Autodesk Inventor part; units mm, degrees
ref_plane "YZ Plane" through (0, 0, 0) normal (1, 0, 0) x (0, 1, 0)
ref_plane "XZ Plane" through (0, 0, 0) normal (0, 1, 0) x (-1, 0, 0)
ref_plane "XY Plane" through (0, 0, 0) normal (0, 0, 1) x (1, 0, 0)
sketch "Sketch1" plane through (0, 0, 0) normal (0, 0, 1) x (1, 0, 0)
  line L0 (0, 0) -> (14.9, 0)
  line L1 (14.9, 0) -> (14.9, 2.75)
  line L2 (14.9, 2.75) -> (12, 2.75)
  line L3 (0, 0) -> (0, 1.5)
  line L4 (0, 1.5) -> (12, 1.5)
  line L5 (12, 1.5) -> (12, 2.75)
  dimension "d0" = 14.9
  dimension "d1" = 2.75
  dimension "d2" = 2.9
  dimension "d3" = 1.5
revolve "Revolution1" add sketch "Sketch1" angle 360 about axis through (0, 0, 0) along (1, 0, 0)
sketch "Sketch2" plane through (14.9, 0, 0) normal (1, 0, 0) x (0, 0, -1)
  line L0 (0.7, 1.2124) -> (1.4, 0)
  line L1 (1.4, 0) -> (0.7, -1.2124)
  line L2 (0.7, -1.2124) -> (-0.7, -1.2124)
  line L3 (-0.7, -1.2124) -> (-1.4, 0)
  line L4 (-1.4, 0) -> (-0.7, 1.2124)
  line L5 (-0.7, 1.2124) -> (0.7, 1.2124)
  point P0 (0, 0)
  point P1 (0, 0)
  dimension "d6" = 2.8
extrude "Extrusion1" cut sketch "Sketch2" against normal blind 1.9
thread "Thread1"
properties part number "fasten_bolt" material "Steel, Mild"
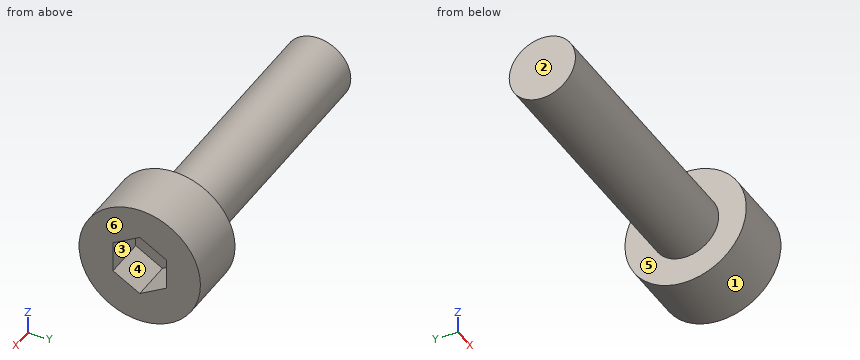
Geometry check sheet. Reference: the model listing, model coordinates, mm. Face numbers are marked on the shaded views. A direction names the side the tool comes from. Give positions to 0.01 mm unless a question says otherwise; leave off trailing zeros. Loops run counter-clockwise (first coordinate to the right, second up) from the corner with the lowest first, then second, coordinate; pieces in that order, holes last.
(1) Section check A-A on x = 13.5. Record the cut outline in (y, z), then the cut area to 3 significant figures.
From the geometry:
outline: circle Ø5.5 at (0, 0); hole (-1.21, -0.7) - (0, -1.4) - (1.21, -0.7) - (1.21, 0.7) - (0, 1.4) - (-1.21, 0.7) - close
area: 18.7 mm2
(2) Set-up check for the marked faces 5 and 6: record each of +Z, -Z, +X, -X, +Y, -Y from which the full face is reachable in a straight line by a thin tool's end or side.
From the geometry:
face 5: -X
face 6: +Z, -Z, +X, +Y, -Y
(3) Section check D-D on x = 5.75. Record the cut outline in (y, z).
From the geometry:
outline: circle Ø3 at (0, 0)
(4) Depth check by flat-ended pin: pin 1 Ø1.2 at (y, z) = (-0.5, 0) entering from +X; pin 2 Ø2 at (x, z) = (12, -1.5) entering from +Y. Enter the tip coordinate at first touch or a pass-through.
From the geometry:
pin 1: stops at x = 13
pin 2: stops at y = 2.7
(5) Thickness scan on L1, parallel to Y at x = 14.25, z = -0.1; L2, parallel to X at y = 0.85, z = -0.25; L3, parallel to X at y = 0.95, z = 1.35. Record the ranges inside material, lowest first.
From the geometry:
L1: y = -2.75 to -1.21, 1.21 to 2.75
L2: x = 0 to 13
L3: x = 12 to 14.9
(6) Section check B-B on z = 0. Record the cut outline in (x, y), then the cut area to 3 significant figures.
From the geometry:
outline: (0, -1.5) - (12, -1.5) - (12, -2.75) - (14.9, -2.75) - (14.9, -1.21) - (13, -1.21) - (13, 1.21) - (14.9, 1.21) - (14.9, 2.75) - (12, 2.75) - (12, 1.5) - (0, 1.5) - close
area: 47.3 mm2
(7) Section check C-C on y = 0.35. Record the cut outline in (x, z).
From the geometry:
outline: (0, -1.46) - (12, -1.46) - (12, -2.73) - (14.9, -2.73) - (14.9, -1.2) - (13, -1.2) - (13, 1.2) - (14.9, 1.2) - (14.9, 2.73) - (12, 2.73) - (12, 1.46) - (0, 1.46) - close
(8) Release check for a two-part mould opening along Z. For the marked faces 1, 2, 3 and 4 record: released by +Z, released by -Z, zero draft, split by the parting line, or undercut.
From the geometry:
face 1: split by the parting line
face 2: zero draft
face 3: undercut
face 4: undercut
